Model file for the job. Use its own axes, mm. Round coordinates to 2 decimals unless told otherwise and drop trailing zeros. Write each loop counter-clockwise with the first axis right and the second up, starting at its lowest first coordinate (ties: lowest second). Pieces come first, ordered by that corner, then holes. Notation, with made-up numbers: (67.5, 55) - (108.5, 55) arc R21 ccw to (108.5, 77) - close; hole circle Ø3 at (10, -18.5). An arc over 180 degrees is marked (long way). One line per item, written item: value.
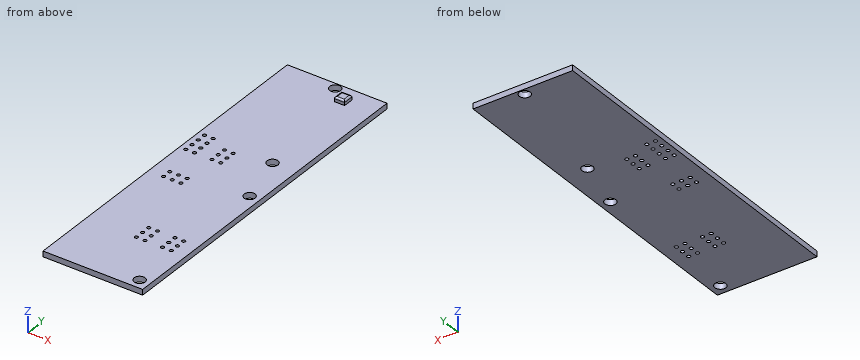
from build123d import *

# Parameters (mm, degrees)
F0_R     = 0.5
F0_R_2   = 1.6
F0_W     = 3
F0_H     = 3
F1_DEPTH = 1.63
F2_DEPTH = 3
F3_R     = 0.5


with BuildPart() as f1:
    # F0 (on Top) → F1 (new body)
    with BuildSketch(Plane.XY):
        Polygon((14.5, -50), (14.5, 50), (-14.5, 50), (-14.5, -50), (-2.65, -50), (7.25, -50), align=None)
        with Locations((-10.13, -6.82)):
            Circle(F0_R, mode=Mode.SUBTRACT)
        with Locations((-7.59, -6.82)):
            Circle(F0_R, mode=Mode.SUBTRACT)
        with Locations((-10.13, -4.28)):
            Circle(F0_R, mode=Mode.SUBTRACT)
        with Locations((-7.59, -4.28)):
            Circle(F0_R, mode=Mode.SUBTRACT)
        with Locations((-5.05, -6.82)):
            Circle(F0_R, mode=Mode.SUBTRACT)
        with Locations((-5.05, -4.28)):
            Circle(F0_R, mode=Mode.SUBTRACT)
        with Locations((0.03, -32.22)):
            Circle(F0_R, mode=Mode.SUBTRACT)
        with Locations((2.57, -32.22)):
            Circle(F0_R, mode=Mode.SUBTRACT)
        with Locations((0.03, -29.68)):
            Circle(F0_R, mode=Mode.SUBTRACT)
        with Locations((0.03, -27.14)):
            Circle(F0_R, mode=Mode.SUBTRACT)
        with Locations((2.57, -29.68)):
            Circle(F0_R, mode=Mode.SUBTRACT)
        with Locations((2.57, -27.14)):
            Circle(F0_R, mode=Mode.SUBTRACT)
        with Locations((11.5, -47)):
            Circle(F0_R_2, mode=Mode.SUBTRACT)
        with Locations((7.65, -32.22)):
            Circle(F0_R, mode=Mode.SUBTRACT)
        with Locations((10.19, -32.22)):
            Circle(F0_R, mode=Mode.SUBTRACT)
        with Locations((7.65, -29.68)):
            Circle(F0_R, mode=Mode.SUBTRACT)
        with Locations((7.65, -27.14)):
            Circle(F0_R, mode=Mode.SUBTRACT)
        with Locations((10.19, -29.68)):
            Circle(F0_R, mode=Mode.SUBTRACT)
        with Locations((10.19, -27.14)):
            Circle(F0_R, mode=Mode.SUBTRACT)
        with Locations((11.5, -2)):
            Circle(F0_R_2, mode=Mode.SUBTRACT)
        with Locations((-12.67, 5.88)):
            Circle(F0_R, mode=Mode.SUBTRACT)
        with Locations((-12.67, 8.42)):
            Circle(F0_R, mode=Mode.SUBTRACT)
        with Locations((-12.67, 10.96)):
            Circle(F0_R, mode=Mode.SUBTRACT)
        with Locations((-10.13, 5.88)):
            Circle(F0_R, mode=Mode.SUBTRACT)
        with Locations((-10.13, 8.42)):
            Circle(F0_R, mode=Mode.SUBTRACT)
        with Locations((-10.13, 10.96)):
            Circle(F0_R, mode=Mode.SUBTRACT)
        with Locations((-12.67, 13.5)):
            Circle(F0_R, mode=Mode.SUBTRACT)
        with Locations((-10.13, 13.5)):
            Circle(F0_R, mode=Mode.SUBTRACT)
        with Locations((-5.05, 5.88)):
            Circle(F0_R, mode=Mode.SUBTRACT)
        with Locations((-5.05, 8.42)):
            Circle(F0_R, mode=Mode.SUBTRACT)
        with Locations((-5.05, 10.96)):
            Circle(F0_R, mode=Mode.SUBTRACT)
        with Locations((-2.51, 5.88)):
            Circle(F0_R, mode=Mode.SUBTRACT)
        with Locations((-2.51, 8.42)):
            Circle(F0_R, mode=Mode.SUBTRACT)
        with Locations((-2.51, 10.96)):
            Circle(F0_R, mode=Mode.SUBTRACT)
        with Locations((7.5, 13)):
            Circle(F0_R_2, mode=Mode.SUBTRACT)
        with Locations((0.75, 48.15)):
            Circle(F0_R_2, mode=Mode.SUBTRACT)
        with Locations((5.41, 44.832)):
            Rectangle(F0_W, F0_H, mode=Mode.SUBTRACT)
        with Locations((5.41, 44.832)):
            Rectangle(F0_W, F0_H)
    extrude(amount=F1_DEPTH)

    # F0 (on Top) → F2 (join)
    with BuildSketch(Plane.XY):
        with Locations((5.41, 44.832)):
            Rectangle(F0_W, F0_H)
    extrude(amount=F2_DEPTH)

    # F3
    f3_edges = [f1.edges().sort_by_distance(p)[0] for p in [
        (6.91, 44.832, 3),
        (5.41, 46.332, 3),
        (3.91, 44.832, 3),
        (5.41, 43.332, 3),
    ]]
    fillet(f3_edges, radius=F3_R)


solid = f1.part
1. Wall check: probe 1 along Y at (x, z) = (-5, 1.25); probe 2 along X at (y, z) = (-32.22, 0.7); probe 3 along Y at (x, z) = (-4.75, 0.1). Give the ranges that are in metal, low to high. Write a range as [from, to].
Report:
probe 1: [-50, -7.32], [-6.32, -4.78], [-3.78, 5.38], [6.38, 7.92], [8.92, 10.46], [11.46, 50]
probe 2: [-14.5, -0.47], [0.53, 2.07], [3.07, 7.15], [8.15, 9.69], [10.69, 14.5]
probe 3: [-50, -7.22], [-6.42, -4.68], [-3.88, 5.48], [6.28, 8.02], [8.82, 10.56], [11.36, 50]
2. Drop flat-ended pins along their axis: pin 1 (8 mm diameter, centred on x = -4, y = -1.5, fed in from +Z); pin 2 (2.5 mm diameter, centred on x = 11.5, y = -2, fed in from +Z). Give the stop position or say it passes through.
Report:
pin 1: z = 1.63
pin 2: through
3. Band-saw the part on A-A on z = 1.1. State how many separate pieces and enclosed holes the cut face has, plus the area to 3 significant figures.
Report:
separate pieces: 1
enclosed holes: 36
area: 2,840 mm²
4. Band-saw the part on B-B on y = -24.5. Write the cut outline in (x, z).
Report:
outline: (-14.5, 0) - (14.5, 0) - (14.5, 1.63) - (-14.5, 1.63) - close
